Input: part model. Units: mm. Frame: model coordinates. A direction names the side the tool comes from. Coordinates: 2 decimals unless noted, no trailing zeros. Order: outer loops, then holes, each group sorted by start corner. A loop starts at its lowest first (then second) coordinate and runs counter-clockwise, first axis right, second up. Notation, with made-up numbers: (58, 77.25) -> (73, 77.25) arc R27 cw to (73, 97.25) -> close; hole circle Ø9 at (9.25, 4.25). An arc over 180 degrees is marked (long way). Use one line per item in the form item = value. Start each with the question number.
1) Ray query, line 1 along Y through (x, z) = (105, 3.2); line 2 along Y through (x, z) = (0, 4.3); line 3 along Y through (x, z) = (-35, 2.55). Return the intervals inside material, ascending.
2) Section query B-B on z = 1.1. Output: boundary loops of the cut face in (x, y), then the cut area to 3 significant figures.
3) Draft query along X for faces 1 (the flat face through (-62, 40, 2)), 2 (the flat face through (115, -1, 2)), 3 (the cylindrical face through (100.754, -29.813, 2.465)), 4 (the flat face through (-115, 1, 2)). Return one class per face: pulls with the +X half, pulls with the -X half, needs draft (parallel to the pull), parting line crosses it, or undercut.
4) Access query for faces 5 (the cylindrical face through (-109.246, 30.187, 2.465)), 6 (the flat face through (10, 38, 2)), 7 (the flat face through (-5, -2, 2)). Directions: +Z, -Z, +X, -X, +Y, -Y. A direction counts if a zero-diameter tool reaches every point of the face in a straight line with its end or side. Return the directions, or none.
5) Section query D-D on x = -105. Output: boundary loops of the cut face in (y, z).
6) Section query A-A on x = -35. Output: boundary loops of the cut face in (y, z), then the cut area to 3 significant figures.
7) Section query C-C on y = 0. Output: boundary loops of the cut face in (x, z), then the cut area to 3 significant figures.
8) Pin query (flat end, axial travel): pin 1 (12 mm diameter, centred on x = 0, y = 0, fed in from -Z); pin 2 (5 mm diameter, centred on x = -105, y = 30, fed in from +Z). Return the tip coordinate at first contact, or that it passes through.
from build123d import *

# Parameters (mm, degrees)
F0_R     = 4.25
F0_R_2   = 9
F0_R_3   = 5
F1_DEPTH = 5
F2_R     = 10
F3_DEPTH = 2


with BuildPart() as f1:
    # F0 (on Top) → F1 (new body)
    with BuildSketch(Plane.XY):
        with BuildLine():
            Line((115, -40), (115, 40))
            Line((115, 40), (10, 40))
            Line((10, 40), (10, 35))
            ThreePointArc((10, 35), (0, 25), (-10, 35))
            Line((-10, 35), (-10, 40))
            Line((-10, 40), (-115, 40))
            Line((-115, 40), (-115, -40))
            Line((-115, -40), (115, -40))
        make_face()
        with Locations((-105, -30)):
            Circle(F0_R, mode=Mode.SUBTRACT)
        with Locations((105, -30)):
            Circle(F0_R, mode=Mode.SUBTRACT)
        with Locations((-35, 0)):
            Circle(F0_R_2, mode=Mode.SUBTRACT)
        with Locations((-105, 30)):
            Circle(F0_R, mode=Mode.SUBTRACT)
        Circle(F0_R_3, mode=Mode.SUBTRACT)
        with Locations((35, 0)):
            Circle(F0_R_2, mode=Mode.SUBTRACT)
        with Locations((105, 30)):
            Circle(F0_R, mode=Mode.SUBTRACT)
    extrude(amount=F1_DEPTH)

    # F2 (on face) → F3 (cut)
    with BuildSketch(Plane.XY):
        Circle(F2_R)
    extrude(amount=F3_DEPTH, mode=Mode.SUBTRACT)


solid = f1.part
Answers below:
q1.line_1 = -40 to -34.25, -25.75 to 25.75, 34.25 to 40
q1.line_2 = -40 to -5, 5 to 25
q1.line_3 = -40 to -9, 9 to 40
q2.outline = (-115, -40) -> (115, -40) -> (115, 40) -> (10, 40) -> (10, 35) arc R10 cw to (-10, 35) -> (-10, 40) -> (-115, 40) -> close; hole circle Ø8.5 at (-105, -30); hole circle Ø8.5 at (-105, 30); hole circle Ø18 at (-35, 0); hole circle Ø20 at (0, 0); hole circle Ø18 at (35, 0); hole circle Ø8.5 at (105, -30); hole circle Ø8.5 at (105, 30)
q2.area = 17,100 mm^2
q3.face_1 = needs draft
q3.face_2 = pulls with the +X half
q3.face_3 = undercut
q3.face_4 = pulls with the -X half
q4.face_5 = +Z, -Z
q4.face_6 = +Z, -Z, +Y
q4.face_7 = -Z
q5.outline = (-40, 0) -> (-34.25, 0) -> (-34.25, 5) -> (-40, 5) -> close; (-25.75, 0) -> (25.75, 0) -> (25.75, 5) -> (-25.75, 5) -> close; (34.25, 0) -> (40, 0) -> (40, 5) -> (34.25, 5) -> close
q6.outline = (-40, 0) -> (-9, 0) -> (-9, 5) -> (-40, 5) -> close; (9, 0) -> (40, 0) -> (40, 5) -> (9, 5) -> close
q6.area = 310 mm^2
q7.outline = (-115, 0) -> (-44, 0) -> (-44, 5) -> (-115, 5) -> close; (-26, 0) -> (-10, 0) -> (-10, 2) -> (-5, 2) -> (-5, 5) -> (-26, 5) -> close; (5, 2) -> (10, 2) -> (10, 0) -> (26, 0) -> (26, 5) -> (5, 5) -> close; (44, 0) -> (115, 0) -> (115, 5) -> (44, 5) -> close
q7.area = 900 mm^2
q8.pin_1 = 2
q8.pin_2 = through
